Model file for the job. Use its own axes, mm. Round coordinates to 2 decimals unless told otherwise and drop trailing zeros. Loops run counter-clockwise (first coordinate to the right, second up) from the corner with the lowest first, then second, coordinate; pieces in that order, holes last. Notation, with made-up numbers: (41, -25.5) - (71, -25.5) arc R31 cw to (71, 13.5) - close; hole circle Ø2 at (55, 56.25). An arc over 180 degrees is marked (long way). Answer as a JSON object with one key per item and string values.
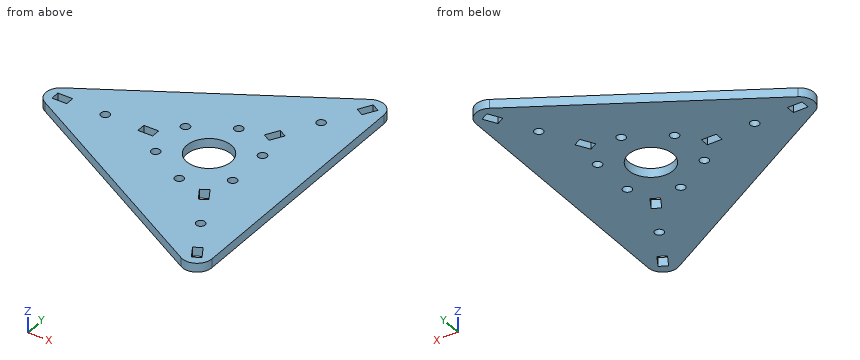
from build123d import *

# Parameters (mm, degrees)
F0_W     = 5
F0_H     = 3
F0_R     = 1.5
F0_R_2   = 7.5
F1_DEPTH = 1.5


with BuildPart() as f1:
    # F0 (on Top) → F1 (new body, symmetric)
    with BuildSketch(Plane.XY):
        with BuildLine():
            Line((22.5, 47.6313972081), (-52.5, 4.3301270189))
            ThreePointArc((-52.5, 4.3301270189), (-55, 0), (-52.5, -4.3301270189))
            Line((-52.5, -4.3301270189), (22.5, -47.6313972081))
            ThreePointArc((22.5, -47.6313972081), (27.5, -47.6313972081), (30, -43.3012701892))
            Line((30, -43.3012701892), (30, 43.3012701892))
            ThreePointArc((30, 43.3012701892), (27.5, 47.6313972081), (22.5, 47.6313972081))
        make_face()
        with Locations((-49.5, 0)):
            Rectangle(F0_W, F0_H, mode=Mode.SUBTRACT)
        with Locations((-35, 0)):
            Circle(F0_R, mode=Mode.SUBTRACT)
        with Locations((-12.9903810568, -7.5)):
            Circle(F0_R, mode=Mode.SUBTRACT)
        with Locations((-20.5, 0)):
            Rectangle(F0_W, F0_H, mode=Mode.SUBTRACT)
        Polygon((22.2009618943, -41.4531939779), (24.7990381057, -39.9531939779), (27.2990381057, -44.2833209968), (24.7009618943, -45.7833209968), align=None, mode=Mode.SUBTRACT)
        with Locations((17.5, -30.3108891325)):
            Circle(F0_R, mode=Mode.SUBTRACT)
        with Locations((0, -15)):
            Circle(F0_R, mode=Mode.SUBTRACT)
        Circle(F0_R_2, mode=Mode.SUBTRACT)
        Polygon((10.2009618943, -20.668584287), (7.7009618943, -16.3384572681), (10.2990381057, -14.8384572681), (12.7990381057, -19.168584287), align=None, mode=Mode.SUBTRACT)
        with Locations((12.9903810568, -7.5)):
            Circle(F0_R, mode=Mode.SUBTRACT)
        with Locations((-12.9903810568, 7.5)):
            Circle(F0_R, mode=Mode.SUBTRACT)
        with Locations((0, 15)):
            Circle(F0_R, mode=Mode.SUBTRACT)
        with Locations((12.9903810568, 7.5)):
            Circle(F0_R, mode=Mode.SUBTRACT)
        Polygon((12.7990381057, 19.168584287), (10.2990381057, 14.8384572681), (7.7009618943, 16.3384572681), (10.2009618943, 20.668584287), align=None, mode=Mode.SUBTRACT)
        with Locations((17.5, 30.3108891325)):
            Circle(F0_R, mode=Mode.SUBTRACT)
        Polygon((24.7990381057, 39.9531939779), (22.2009618943, 41.4531939779), (24.7009618943, 45.7833209968), (27.2990381057, 44.2833209968), align=None, mode=Mode.SUBTRACT)
    extrude(amount=F1_DEPTH, both=True)


solid = f1.part
1) Slice it at A-A on y = 0. List the corners of the cut face in (x, z).
Values follow:
{"outline": "(-55, -1.5) - (-52, -1.5) - (-52, 1.5) - (-55, 1.5) - close; (-47, -1.5) - (-36.5, -1.5) - (-36.5, 1.5) - (-47, 1.5) - close; (-33.5, -1.5) - (-23, -1.5) - (-23, 1.5) - (-33.5, 1.5) - close; (-18, -1.5) - (-7.5, -1.5) - (-7.5, 1.5) - (-18, 1.5) - close; (7.5, -1.5) - (30, -1.5) - (30, 1.5) - (7.5, 1.5) - close"}
2) Probe probe 1 along Y at (x, z) = (0, -0.05); probe 2 along Y at (x, z) = (26, -0.35); probe 3 along Y at (x, z) = (24, 1.05). List the from-to ranges inside material, lowest first.
Values follow:
{"probe 1": "-34.64 to -16.5, -13.5 to -7.5, 7.5 to 13.5, 16.5 to 34.64", "probe 2": "-48.2 to -45.03, -42.03 to 42.03, 45.03 to 48.2", "probe 3": "-48.2 to -44.57, -40.41 to 40.41, 44.57 to 48.2"}
3) Slice it at D-D on x = 17.5. List the corners of the cut face in (y, z), then the cut area to 3 significant figures.
Values follow:
{"outline": "(-44.74, -1.5) - (-31.81, -1.5) - (-31.81, 1.5) - (-44.74, 1.5) - close; (-28.81, -1.5) - (28.81, -1.5) - (28.81, 1.5) - (-28.81, 1.5) - close; (31.81, -1.5) - (44.74, -1.5) - (44.74, 1.5) - (31.81, 1.5) - close", "area": "250 mm²"}
4) Slice it at C-C on x = -35. List the corners of the cut face in (y, z), then the cut area to 3 significant figures.
Values follow:
{"outline": "(-14.43, -1.5) - (-1.5, -1.5) - (-1.5, 1.5) - (-14.43, 1.5) - close; (1.5, -1.5) - (14.43, -1.5) - (14.43, 1.5) - (1.5, 1.5) - close", "area": "77.6 mm²"}
5) Drop flat-ended pins along their axis: P1, Ø4, axis at x = 17.5, y = -30.31, coming from the -Z side; P2, Ø0.9, axis at x = -19.5, z = -0.5, coming from the -Y side. Give the stop position or say it passes through.
Values follow:
{"P1": "z = -1.5", "P2": "y = -23.64"}
6) Slice it at B-B on x = 0. List the corners of the cut face in (y, z), then the cut area to 3 significant figures.
Values follow:
{"outline": "(-34.64, -1.5) - (-16.5, -1.5) - (-16.5, 1.5) - (-34.64, 1.5) - close; (-13.5, -1.5) - (-7.5, -1.5) - (-7.5, 1.5) - (-13.5, 1.5) - close; (7.5, -1.5) - (13.5, -1.5) - (13.5, 1.5) - (7.5, 1.5) - close; (16.5, -1.5) - (34.64, -1.5) - (34.64, 1.5) - (16.5, 1.5) - close", "area": "145 mm²"}
